Here's how the part is built. I have some questions about the finished solid (model axes, mm). A direction names the side the tool comes from. Coordinates: 2 decimals unless noted, no trailing zeros. Loops run counter-clockwise (first coordinate to the right, second up) from the corner with the lowest first, then second, coordinate; pieces in that order, holes last.
```python
from build123d import *

# Parameters (mm, degrees)
SKETCH1_W           = 120
SKETCH1_H           = 90
BOSS_EXTRUDE1_DEPTH = 3
SKETCH3_R           = 1.75
SKETCH3_R_2         = 1.05
CUT_EXTRUDE1_DEPTH  = 3
SKETCH7_R           = 1.25
CUT_EXTRUDE3_DEPTH  = 3


with BuildPart() as part:
    # Sketch1 → Boss-Extrude1 (new body)
    with BuildSketch(Plane.XY):
        with Locations((60, -45)):
            Rectangle(SKETCH1_W, SKETCH1_H)
    extrude(amount=BOSS_EXTRUDE1_DEPTH)

    # Sketch3 → Cut-Extrude1 (cut)
    with BuildSketch(Plane.XY.offset(3)):
        with Locations((24, -44.9)):
            Circle(SKETCH3_R)
        with Locations((80.856366148, -63.762627499)):
            Circle(SKETCH3_R_2)
        with BuildLine():
            Line((79.806366148, -29.090746885), (79.806366148, -21.14956271))
            ThreePointArc((79.806366148, -21.14956271), (80.856366148, -20.09956271), (81.906366148, -21.14956271))
            Line((81.906366148, -21.14956271), (81.906366148, -29.090746885))
            ThreePointArc((81.906366148, -29.090746885), (80.856366148, -30.140746885), (79.806366148, -29.090746885))
        make_face()
    extrude(amount=-CUT_EXTRUDE1_DEPTH, mode=Mode.SUBTRACT)

    # Sketch7 → Cut-Extrude3 (cut)
    with BuildSketch(Plane.XY.offset(3)):
        with Locations((80.856366148, -15.59956271)):
            Circle(SKETCH7_R)
        with Locations((87.870361331, -7.785865021)):
            Circle(SKETCH7_R)
    extrude(amount=-CUT_EXTRUDE3_DEPTH, mode=Mode.SUBTRACT)


solid = part.part
```
1. On a 3-axis mill with a long thin cutter (end or side, diameter ignored), from which of +Z, -Z, +X, -X, +Y, -Y can I reach the whole of each face in a straight line? I mean faces 5 (the flat face through (81.906, -25, 2)), 6 (the flat face through (0, -46, 1)). Say none if no direction works.
2. I want a section at B-B (x = 24). Please give me the cut outline in (y, z), then the cut area to 4 significant figures.
3. I want a section at A-A (y = -44.9). Please give me the cut outline in (x, z), then the cut area to 4 significant figures.
4. We'd pull the mould along Y, two halves only. Please class faces 1 (the flat face through (59, 0, 1)), 2 (the cylindrical face through (22.61, -45.96, 1.52)), 3 (the flat face through (59, -44, 0)), 4 (the flat face through (59, -90, 1)): +Y half, -Y half, draft (parallel to the pull), parting line (faces both ways), or undercut.
5. I need wall thicknesses on line 1 along Y through (x, z) = (24, 0.6); line 2 along X through (y, z) = (-44, 0.85); line 3 along X through (y, z) = (-43.5, 0.65). Which ranges of each line are inside material? Lowest first, please.
Response values:
1. face 5: +Z, -Z
1. face 6: +Z, -Z, -X, +Y, -Y
2. outline: (-90, 0) - (-46.65, 0) - (-46.65, 3) - (-90, 3) - close; (-43.15, 0) - (0, 0) - (0, 3) - (-43.15, 3) - close
2. area: 259.5 mm2
3. outline: (0, 0) - (22.25, 0) - (22.25, 3) - (0, 3) - close; (25.75, 0) - (120, 0) - (120, 3) - (25.75, 3) - close
3. area: 349.5 mm2
4. face 1: +Y half
4. face 2: undercut
4. face 3: draft
4. face 4: -Y half
5. line 1: y = -90 to -46.65, -43.15 to 0
5. line 2: x = 0 to 22.5, 25.5 to 120
5. line 3: x = 0 to 22.95, 25.05 to 120
